Work out the finished part from the listing and answer in its coordinate system (mm). Face numbers are marked on the shaded views. Coordinates: 2 decimals unless noted, no trailing zeros. Order: outer loops, then holes, each group sorted by start corner. A loop starts at its lowest first (then second) coordinate and runs counter-clockwise, first axis right, second up. Notation, with made-up numbers: (82, 0.25) -> (125, 0.25) arc R12 cw to (125, 23.25) -> close; hole circle Ø6 at (61.25, -25.75). An arc over 180 degrees is marked (long way). Use one line per item in the form item = value.
from build123d import *

# Parameters (mm, degrees)
F0_W      = 209.55
F0_H      = 52.07
F0_R      = 1.905
F1_DEPTH  = 2.999994
F3_DEPTH  = 2.999994
F4_R      = 1.397
F5_DEPTH  = 25.4
F6_R      = 3.6195
F6_R_2    = 1.397
F7_DEPTH  = 3.5052
F8_SIZE   = 1.143
F10_DEPTH = 25.4


with BuildPart() as f1:
    # F0 (on Top) → F1 (new body)
    with BuildSketch(Plane.XY):
        with Locations((-104.775, -26.035)):
            Rectangle(F0_W, F0_H)
        with Locations((-205.24089, -46.99)):
            Circle(F0_R, mode=Mode.SUBTRACT)
        with Locations((-4.30911, -46.99)):
            Circle(F0_R, mode=Mode.SUBTRACT)
        with Locations((-205.24089, -5.08)):
            Circle(F0_R, mode=Mode.SUBTRACT)
        with Locations((-4.30911, -5.08)):
            Circle(F0_R, mode=Mode.SUBTRACT)
    extrude(amount=F1_DEPTH)

    # F2 (on face) → F3 (join, through all)
    with BuildSketch(Plane.XY.offset(2.999994)):
        Polygon((-56.0324, -52.07), (-163.8554, -52.07), (-150.9903, -64.924351), (-68.8975, -64.924351), align=None)
    extrude(amount=-F3_DEPTH)

    # F4 (on face) → F5 (cut)
    with BuildSketch(Plane.XY.offset(2.999994)):
        with Locations((-70.993, -12.6238)):
            Circle(F4_R)
        with BuildLine():
            ThreePointArc((-71.980828, -59.921372), (-71.527609, -62.19986), (-69.596, -60.9092))
            ThreePointArc((-69.596, -60.9092), (-70.458391, -59.61854), (-71.980828, -59.921372))
        make_face()
        with BuildLine():
            ThreePointArc((-120.406289, -45.660725), (-120.512629, -45.126116), (-120.815461, -44.672897))
            ThreePointArc((-120.815461, -44.672897), (-123.093949, -46.195334), (-120.406289, -45.660725))
        make_face()
        with Locations((-153.543, -12.6238)):
            Circle(F4_R)
        with Locations((-145.923, -60.9092)):
            Circle(F4_R)
        with Locations((-121.803289, -17.720725)):
            Circle(F4_R)
    extrude(amount=-F5_DEPTH, mode=Mode.SUBTRACT)

    # F6 (on face) → F7 (join)
    with BuildSketch(Plane.XY.offset(2.999994)):
        with Locations((-153.543, -12.6238)):
            Circle(F6_R)
        with Locations((-153.543, -12.6238)):
            Circle(F6_R_2, mode=Mode.SUBTRACT)
        with Locations((-145.923, -60.9092)):
            Circle(F6_R)
        with Locations((-145.923, -60.9092)):
            Circle(F6_R_2, mode=Mode.SUBTRACT)
        with Locations((-121.803289, -45.660725)):
            Circle(F6_R)
        with Locations((-121.803289, -45.660725)):
            Circle(F6_R_2, mode=Mode.SUBTRACT)
        with Locations((-121.803289, -17.720725)):
            Circle(F6_R)
        with Locations((-121.803289, -17.720725)):
            Circle(F6_R_2, mode=Mode.SUBTRACT)
        with Locations((-70.993, -12.6238)):
            Circle(F6_R)
        with Locations((-70.993, -12.6238)):
            Circle(F6_R_2, mode=Mode.SUBTRACT)
        with Locations((-70.993, -60.9092)):
            Circle(F6_R)
        with Locations((-70.993, -60.9092)):
            Circle(F6_R_2, mode=Mode.SUBTRACT)
    extrude(amount=F7_DEPTH)

    # F8
    f8_edges = [f1.edges().sort_by_distance(p)[0] for p in [
        (-157.1625, -12.6238, 6.505194),
        (-125.422789, -17.720725, 6.505194),
        (-125.422789, -45.660725, 6.505194),
        (-149.5425, -60.9092, 6.505194),
        (-74.6125, -60.9092, 6.505194),
        (-74.6125, -12.6238, 6.505194),
    ]]
    chamfer(f8_edges, length=F8_SIZE)

    # F9 (on face) → F10 (cut)
    with BuildSketch(Plane.XY.offset(2.999994)):
        with BuildLine():
            ThreePointArc((-15.24, -15.24), (-16.727898, -11.647898), (-20.32, -10.16))
            Line((-20.32, -10.16), (-51.095472, -10.16))
            ThreePointArc((-51.095472, -10.16), (-54.687574, -11.647898), (-56.175472, -15.24))
            Line((-56.175472, -15.24), (-56.175472, -16.951881))
            ThreePointArc((-56.175472, -16.951881), (-57.663369, -20.543983), (-61.255472, -22.031881))
            Line((-61.255472, -22.031881), (-104.023289, -22.031881))
            ThreePointArc((-104.023289, -22.031881), (-107.615392, -23.519778), (-109.103289, -27.111881))
            Line((-109.103289, -27.111881), (-109.103289, -36.83))
            ThreePointArc((-109.103289, -36.83), (-107.615392, -40.422102), (-104.023289, -41.91))
            Line((-104.023289, -41.91), (-56.175472, -41.91))
            Line((-56.175472, -41.91), (-20.32, -41.91))
            ThreePointArc((-20.32, -41.91), (-16.727898, -40.422102), (-15.24, -36.83))
            Line((-15.24, -36.83), (-15.24, -15.24))
        make_face()
        with BuildLine():
            Line((-175.018272, -10.16), (-189.23, -10.16))
            ThreePointArc((-189.23, -10.16), (-192.822102, -11.647898), (-194.31, -15.24))
            Line((-194.31, -15.24), (-194.31, -36.83))
            ThreePointArc((-194.31, -36.83), (-192.822102, -40.422102), (-189.23, -41.91))
            Line((-189.23, -41.91), (-169.938272, -41.91))
            Line((-169.938272, -41.91), (-139.583289, -41.91))
            ThreePointArc((-139.583289, -41.91), (-135.991187, -40.422102), (-134.503289, -36.83))
            Line((-134.503289, -36.83), (-134.503289, -27.111881))
            ThreePointArc((-134.503289, -27.111881), (-135.991187, -23.519778), (-139.583289, -22.031881))
            Line((-139.583289, -22.031881), (-164.858272, -22.031881))
            ThreePointArc((-164.858272, -22.031881), (-168.450374, -20.543983), (-169.938272, -16.951881))
            Line((-169.938272, -16.951881), (-169.938272, -15.24))
            ThreePointArc((-169.938272, -15.24), (-171.426169, -11.647898), (-175.018272, -10.16))
        make_face()
    extrude(amount=-F10_DEPTH, mode=Mode.SUBTRACT)


solid = f1.part
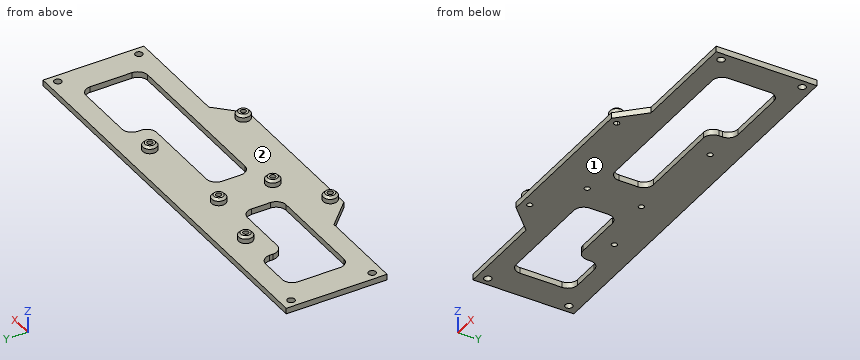
(1) Each of these flat-tipped pins is pushed along its axis until it touches: P1, Ø2, axis at y = -46, z = 5, coming from the +X side; P2, Ø3, axis at x = -205.24, y = -46.99, coming from the -Z side; P3, Ø6, axis at x = -4.31, y = -46.99, coming from the +Z side; P4, Ø2.5, axis at x = -179, z = 1, coming from the -Y side. Where does it stop, or does it pass through?
Data:
P1 = -118.18
P2 = through
P3 = 3
P4 = -52.07
(2) Section A-A on x = -99.5 is taken. Write down the section's boundary in (y, z), plus the area to 3 significant figures.
Data:
outline = (-64.92, 0) -> (-41.91, 0) -> (-41.91, 3) -> (-64.92, 3) -> close; (-22.03, 0) -> (0, 0) -> (0, 3) -> (-22.03, 3) -> close
area = 135 mm²
(3) Straight lines are drawn through the part: line 1 along X through (y, z) = (-18, 3.25); line 2 along Y through (x, z) = (-32, 1); line 3 along Z through (x, y) = (-69, -4.5). For each, find the intervals that lie inside material, in ascending order.
Data:
line_1 = -125.41 to -123.17, -120.43 to -118.19
line_2 = -52.07 to -41.91, -10.16 to 0
line_3 = 0 to 3
(4) The mould has two halves that part along X. Classify the marked faces 1 and 2: released by +X, released by -X, zero draft, split by the parting line, or undercut.
Data:
face_1 = zero draft
face_2 = undercut
(5) Section B-B on y = -5.08 is taken. Write down the section's boundary in (x, z), plus the area to 3 significant figures.
Data:
outline = (-209.55, 0) -> (-207.15, 0) -> (-207.15, 3) -> (-209.55, 3) -> close; (-203.34, 0) -> (-6.21, 0) -> (-6.21, 3) -> (-203.34, 3) -> close; (-2.4, 0) -> (0, 0) -> (0, 3) -> (-2.4, 3) -> close
area = 606 mm²
(6) Section C-C on x = -33.5 is taken. Write down the section's boundary in (y, z), plus the area to 3 significant figures.
Data:
outline = (-52.07, 0) -> (-41.91, 0) -> (-41.91, 3) -> (-52.07, 3) -> close; (-10.16, 0) -> (0, 0) -> (0, 3) -> (-10.16, 3) -> close
area = 61.0 mm²
(7) Section D-D on x = -129.5 is taken. Write down the section's boundary in (y, z).
Data:
outline = (-64.92, 0) -> (0, 0) -> (0, 3) -> (-64.92, 3) -> close
